from build123d import *

# Parameters (mm, degrees)
EXTRUDE_1_DEPTH   = 2
HOLE_WIZARD_M81_D = 9
CHAMFER_1_SIZE    = 2


with BuildPart() as part:
    # Эскиз1 → Бобышка-Вытянуть1 (new body)
    with BuildSketch(Plane(origin=(0, 0, 0), x_dir=(1, 0, 0), z_dir=(0, 0, -1))):
        Polygon((0, 0), (0, 135), (135, 135), (135, 90), (45, 0), align=None)
    extrude(amount=EXTRUDE_1_DEPTH)

    # Отверстие с зазором M81 (through all)
    with Locations(Plane(origin=(0, 0, -2), x_dir=(1, 0, 0), z_dir=(0, 0, -1))):
        with Locations((67.5, 112.5), (22.5, 112.5), (22.5, 67.5), (22.5, 22.5), (112.5, 112.5), (67.5, 67.5)):
            Hole(HOLE_WIZARD_M81_D / 2)

    # Фаска1
    chamfer_1_edges = [part.edges().sort_by_distance(p)[0] for p in [
        (0, 0, -1),
        (0, -135, -1),
        (135, -135, -1),
    ]]
    chamfer(chamfer_1_edges, length=CHAMFER_1_SIZE)


solid = part.part
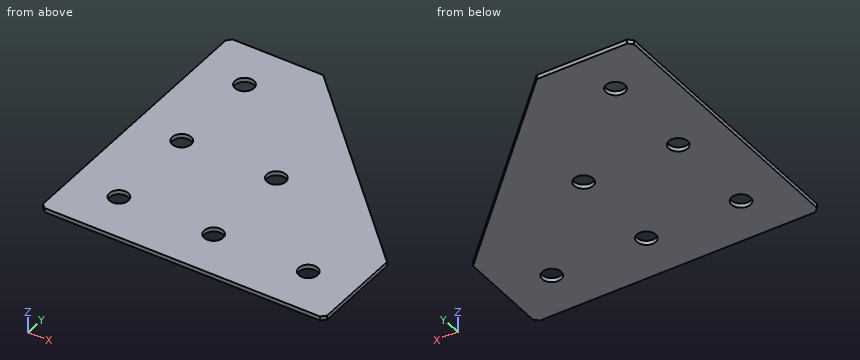
Verification items for the finished model (mm, model axes). Coordinates: 2 decimals unless noted, no trailing zeros. Order: outer loops, then holes, each group sorted by start corner. A loop starts at its lowest first (then second) coordinate and runs counter-clockwise, first axis right, second up. Notation, with made-up numbers: M -28,36 L -9,36 A22 cw -9,43 Z; hole C -31,-38 d8. An arc over 180 degrees is marked long. One line per item, written item: value. Start each with the question number.
Item 1: Sectioned sample at D-D (y = -112.5). Enter the section's corners in (x, z), then the cut area to 3 significant figures.
Item 2: Sectioned sample at C-C (z = -0.45). Enter the section's corners in (x, y).
Item 3: Scan lines: probe 1 along X at (y, z) = (-112.5, -0.8); probe 2 along X at (y, z) = (-67.5, -1.45); probe 3 along Y at (x, z) = (67.5, -1.05). Record each from-to range of solid material in increasing order.
Item 4: Sectioned sample at A-A (x = 67.5). Enter the section's corners in (y, z), then the cut area to 3 significant figures.
Item 5: Sectioned sample at B-B (y = -67.5). Enter the section's corners in (x, z).
Item 6: Gauge pin test, flat end, axial feed: pin 1 (10.5 mm diameter, centred on x = 112.5, y = -112.5, fed in from -Z). Record the tip position at first contact, or that the pin passes through.
Conclusion:
1. outline: M 0,-2 L 18,-2 L 18,0 L 0,0 Z; M 27,-2 L 63,-2 L 63,0 L 27,0 Z; M 72,-2 L 108,-2 L 108,0 L 72,0 Z; M 117,-2 L 135,-2 L 135,0 L 117,0 Z
1. area: 216 mm^2
2. outline: M 0,-133 L 2,-135 L 133,-135 L 135,-133 L 135,-90 L 45,0 L 2,0 L 0,-2 Z; hole C 22.5,-112.5 d9; hole C 22.5,-67.5 d9; hole C 22.5,-22.5 d9; hole C 67.5,-112.5 d9; hole C 67.5,-67.5 d9; hole C 112.5,-112.5 d9
3. probe 1: x = 0 to 18, 27 to 63, 72 to 108, 117 to 135
3. probe 2: x = 0 to 18, 27 to 63, 72 to 112.5
3. probe 3: y = -135 to -117, -108 to -72, -63 to -22.5
4. outline: M -135,-2 L -117,-2 L -117,0 L -135,0 Z; M -108,-2 L -72,-2 L -72,0 L -108,0 Z; M -63,-2 L -22.5,-2 L -22.5,0 L -63,0 Z
4. area: 189 mm^2
5. outline: M 0,-2 L 18,-2 L 18,0 L 0,0 Z; M 27,-2 L 63,-2 L 63,0 L 27,0 Z; M 72,-2 L 112.5,-2 L 112.5,0 L 72,0 Z
6. pin 1: stops at z = -2
